from build123d import *

# Parameters (mm, degrees)
MODEL_R             = 1.575
BOSS_EXTRUDE1_DEPTH = 3
FILLET1_R           = 1


with BuildPart() as part:
    # Model → Boss-Extrude1 (new body)
    with BuildSketch(Plane.XY):
        Polygon((142.344747242, 270.871489374), (153.37187249, 271.263447748), (162.091473536, 274.767362889), (160.85900272, 279.367807803), (179.260689602, 284.297666211), (178.028627015, 288.898354165), (208.019481767, 296.93522173), (209.252454514, 292.334187025), (227.65276755, 297.263677376), (230.276304619, 287.470798216), (275.446186014, 299.571346393), (298.39980436, 213.909597233), (260.87259576, 203.855963236), (255.943287021, 222.255598366), (248.650938057, 220.301667543), (251.115775513, 211.101166572), (220.422247557, 202.878292884), (219.189771603, 207.477473721), (213.081966369, 205.841177268), (214.314693354, 201.241059665), (196.039346948, 196.343682115), (196.007810089, 177.840578221), (186.702312667, 152.27893851), (161.565977706, 161.426447529), (132.435827139, 161.934428279), (107.399642776, 152.824765622), (97.980730454, 178.710864183), (99.858189105, 195.997881416), (81.758593313, 200.846808858), (82.991121062, 205.447466285), (76.882860045, 207.083884844), (75.650856625, 202.485184579), (44.956891994, 210.708175253), (47.421773629, 219.90863481), (40.129543563, 221.862285479), (35.199939127, 203.463086712), (-2.32684459, 213.517448416), (20.785545351, 299.774827661), (65.955825932, 287.671594898), (68.42160019, 296.872525865), (86.820985153, 291.940533454), (88.054439652, 296.542595671), (118.044472643, 288.503706576), (116.812112756, 283.905728394), (135.211333861, 278.973779905), (133.979081507, 274.376202933), align=None)
        with Locations((23.035554, 295.877718337)):
            Circle(MODEL_R, mode=Mode.SUBTRACT)
        with Locations((109.301822433, 156.902965293)):
            Circle(MODEL_R, mode=Mode.SUBTRACT)
        with Locations((184.800560745, 156.35733766)):
            Circle(MODEL_R, mode=Mode.SUBTRACT)
        with Locations((193.847437398, 289.84318413)):
            Circle(MODEL_R, mode=Mode.SUBTRACT)
        with Locations((102.225689846, 289.449650012)):
            Circle(MODEL_R, mode=Mode.SUBTRACT)
        with Locations((273.19609114, 295.674286852)):
            Circle(MODEL_R, mode=Mode.SUBTRACT)
        with Locations((1.570241786, 215.767496811)):
            Circle(MODEL_R, mode=Mode.SUBTRACT)
        with Locations((294.502731407, 216.159668876)):
            Circle(MODEL_R, mode=Mode.SUBTRACT)
        with Locations((80.760413887, 209.339268578)):
            Circle(MODEL_R, mode=Mode.SUBTRACT)
        with Locations((215.312231294, 209.732861073)):
            Circle(MODEL_R, mode=Mode.SUBTRACT)
        Polygon((271.203498451, 292.223209107), (291.05122826, 218.15247975), (265.115556398, 211.204247731), (260.186189629, 229.604099473), (241.30271159, 224.544411578), (243.767491017, 215.34412721), (224.664804007, 210.226469096), (223.432328054, 214.825649934), (205.733277658, 210.084029615), (206.966112962, 205.483507804), (188.744476932, 200.600523414), (190.038361872, 195.770837942), (190.009613349, 178.903688177), (183.116533861, 159.968814913), (162.674398087, 167.40803076), (131.428930231, 167.95289908), (110.986427135, 160.514692668), (104.096364698, 179.45072575), (105.814746135, 195.273012707), (107.149713912, 200.256048118), (89.106877808, 205.089769496), (90.339405557, 209.690426923), (72.639899407, 214.432169339), (71.407895987, 209.833469074), (52.305208977, 214.951127188), (54.770081908, 224.151554257), (35.886712889, 229.210569975), (30.957132238, 210.811459981), (5.0216469, 217.76022363), (25.028202346, 292.426367848), (70.198239559, 280.323200295), (72.663861356, 289.523562363), (91.063082461, 284.591613875), (92.29653696, 289.193676092), (110.695758065, 284.261727603), (109.463398178, 279.663749421), (127.862619282, 274.731800932), (126.630323598, 270.134062294), (145.381260936, 265.108396206), (150.690394167, 265.500431998), (169.439649748, 270.524806438), (168.207287216, 275.124847165), (186.60841776, 280.054556529), (185.376246939, 284.655648642), (203.777033628, 289.586641337), (205.009898064, 284.986010813), (223.409806911, 289.915392881), (226.033325469, 280.122582817), align=None, mode=Mode.SUBTRACT)
    extrude(amount=-BOSS_EXTRUDE1_DEPTH)

    # Fillet1
    fillet1_edges = [part.edges().sort_by_distance(p)[0] for p in [
        (-2.32684459, 213.517448416, -1.5),
        (20.785545351, 299.774827661, -1.5),
        (65.955825932, 287.671594898, -1.5),
        (68.42160019, 296.872525865, -1.5),
        (86.820985153, 291.940533454, -1.5),
        (88.054439652, 296.542595671, -1.5),
        (118.044472643, 288.503706576, -1.5),
        (135.211333861, 278.973779905, -1.5),
        (160.85900272, 279.367807803, -1.5),
        (178.028627015, 288.898354165, -1.5),
        (208.019481767, 296.93522173, -1.5),
        (227.65276755, 297.263677376, -1.5),
        (275.446186014, 299.571346393, -1.5),
        (298.39980436, 213.909597233, -1.5),
        (260.87259576, 203.855963236, -1.5),
        (251.115775513, 211.101166572, -1.5),
        (220.422247557, 202.878292884, -1.5),
        (214.314693354, 201.241059665, -1.5),
        (186.702312667, 152.27893851, -1.5),
        (107.399642776, 152.824765622, -1.5),
        (81.758593313, 200.846808858, -1.5),
        (75.650856625, 202.485184579, -1.5),
        (44.956891994, 210.708175253, -1.5),
        (35.199939127, 203.463086712, -1.5),
    ]]
    fillet(fillet1_edges, radius=FILLET1_R)


solid = part.part
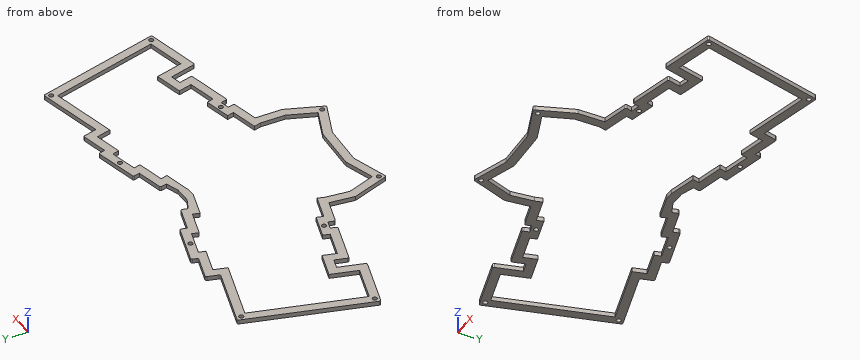
The listing builds one solid part. Answer for the finished solid, in the listing's coordinates (mm). Coordinates: 2 decimals unless noted, no trailing zeros. Order: outer loops, then holes, each group sorted by start corner. A loop starts at its lowest first (then second) coordinate and runs counter-clockwise, first axis right, second up.
Q1. A cutting plane is placed at B-B, the plane x = 199. Write down the section's boundary in (y, z), and give its area (3 significant figures).
Q2. Consider line 1 (X direction, y = 272.5, z = -1.1); line 2 (X direction, y = 223.5, z = -1.8); line 3 (Y direction, x = 216, z = -0.8). Determine where each line is inside the solid, lowest interval first.
Q3. A cutting plane is placed at C-C, the plane z = -1.9. State how many separate pieces and enclosed holes the cut face has, and give its area (3 significant figures).
Q4. Given P1, Ø1, axis at x = 130.5, z = -2.5, coming from the -Y side; P2, Ø3, axis at x = 193.85, y = 289.84, coming from the -Z side, each flat-ended and moving along its own axis, determine where each tip first touches the part or whether it passes through.
Q5. A cutting plane is placed at A-A, the plane y = 190. Write down the section's boundary in (x, z), and give its area (3 significant figures).
Answers follow:
1. outline: (197.14, -3) - (203.35, -3) - (203.35, 0) - (197.14, 0) - close; (288.31, -3) - (294.52, -3) - (294.52, 0) - (288.31, 0) - close
1. area: 37.3 mm2
2. line 1: x = 13.48 to 19.69, 127.26 to 138.46, 156.45 to 168.91, 276.49 to 282.7
2. line 2: x = 0.35 to 6.56, 34.36 to 54.6, 241.58 to 261.82, 289.62 to 295.83
2. line 3: y = 206.62 to 208.32, 211.15 to 212.83, 287.93 to 294.14
3. separate pieces: 1
3. enclosed holes: 11
3. area: 5,410 mm2
4. P1: stops at y = 161.05
4. P2: passes through
5. outline: (99.21, -3) - (105.24, -3) - (105.24, 0) - (99.21, 0) - close; (190.03, -3) - (196.03, -3) - (196.03, 0) - (190.03, 0) - close
5. area: 36.1 mm2
